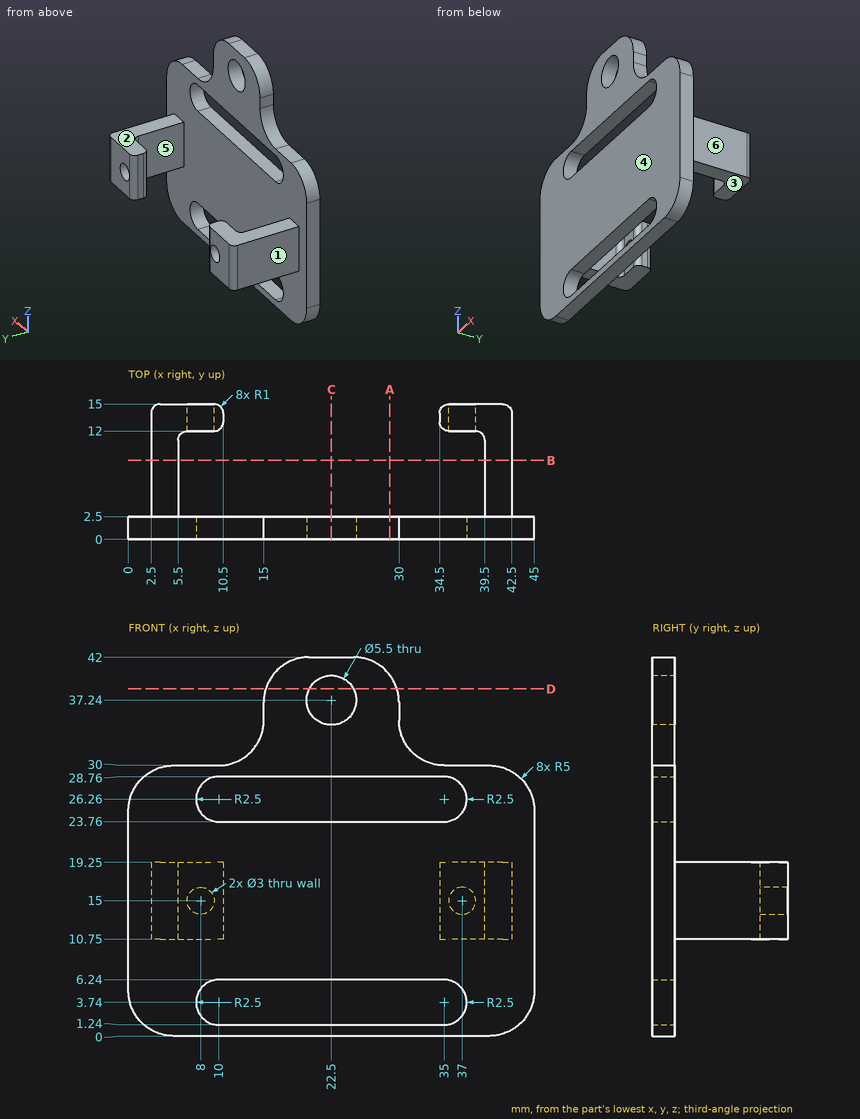
Geometry check sheet. Reference: drawing and pictorial views, mm from the part's lowest x, y, z. A direction names the side the tool comes from. Give positions to 0.01 mm unless a question says otherwise; leave off trailing zeros. Order: outer loops, then holes, each group sorted by start corner. A loop starts at its lowest first (then second) coordinate and runs counter-clockwise, first axis right, second up. Notation, with made-up numbers: M 24,47 L 82,47 A18 cw 82,79 Z; hole C 55.5,41.25 d3. An arc over 180 degrees is marked long. Answer in a Markdown table with one row per item. Add a question column.
Item 1: Gauge pin test, flat ends, axial feed: pin 1 (6 mm diameter, centred on y = 2, z = 11.5, fed in from -X); pin 2 (2.5 mm diameter, centred on x = 8, z = 15, fed in from +Y); pin 3 (5 mm diameter, centred on x = 40, y = 13, fed in from -Z); pin 4 (1.5 mm diameter, centred on y = 5, z = 22, fed in from +X). Record the tip position at first contact, or that the pin passes through.
Item 2: Section check A-A, the plane x = 29. Enter the section's corners in (y, z).
Item 3: Section check B-B, the plane y = 8.75. Enter the section's corners in (x, z).
Item 4: Mould release check, pull along Y, two halves, no side actions. Record for the marked faces 4, 5 and 6: released by +Y, released by -Y, zero draft, split by the parting line, or undercut.
Item 5: Scan lines: probe 1 along Z at (x, y) = (37, 13.2); probe 2 along X at (y, z) = (13.65, 15); probe 3 along X at (y, z) = (1.25, 28.5). Record each from-to range of solid material in increasing order. Write a range as from..to.
Item 6: Tool access check on the marked faces 1, 2 and 3. Record the directions out of +Z, -Z, +X, -X, +Y, -Y that give a thin tool (end or side, any length) a straight path to the whole face; none if there is none.
Item 7: Section check D-D, the plane z = 38.5. Enter the section's corners in (x, y).
Item 8: Section check C-C, the plane x = 22.5. Enter the section's corners in (y, z).
Filled sheet:
| question | item | result |
|---|---|---|
| 1 | pin 1 | stops at x = 0 |
| 1 | pin 2 | stops at y = 2.5 |
| 1 | pin 3 | stops at z = 10.75 |
| 1 | pin 4 | passes through |
| 2 | outline | M 0,0 L 2.5,0 L 2.5,1.24 L 0,1.24 Z; M 0,6.24 L 2.5,6.24 L 2.5,23.76 L 0,23.76 Z; M 0,28.76 L 2.5,28.76 L 2.5,40 L 0,40 Z |
| 3 | outline | M 2.5,10.75 L 5.5,10.75 L 5.5,19.25 L 2.5,19.25 Z; M 39.5,10.75 L 42.5,10.75 L 42.5,19.25 L 39.5,19.25 Z |
| 4 | face 4 | released by -Y |
| 4 | face 5 | undercut |
| 4 | face 6 | zero draft |
| 5 | probe 1 | z = 10.75..13.5, 16.5..19.25 |
| 5 | probe 2 | x = 2.5..6.5, 9.5..10.5, 34.5..35.5, 38.5..42.5 |
| 5 | probe 3 | x = 1.43..8.89, 36.11..43.57 |
| 6 | face 1 | +Z, -Z, -X, +Y |
| 6 | face 2 | +Z, +X, -X, +Y |
| 6 | face 3 | -Z, +X, -X, +Y |
| 7 | outline | M 15.23,0 L 20.06,0 L 20.06,2.5 L 15.23,2.5 Z; M 24.94,0 L 29.77,0 L 29.77,2.5 L 24.94,2.5 Z |
| 8 | outline | M 0,0 L 2.5,0 L 2.5,1.24 L 0,1.24 Z; M 0,6.24 L 2.5,6.24 L 2.5,23.76 L 0,23.76 Z; M 0,28.76 L 2.5,28.76 L 2.5,34.49 L 0,34.49 Z; M 0,39.99 L 2.5,39.99 L 2.5,42 L 0,42 Z |
